Autodesk Inventor part; units mm, degrees
ref_plane "Work Plane1" through (0, -29.2355, 5.6836) normal (0, 0, 1) x (1, 0, 0)
ref_plane "Work Plane2" through (8.9574, 21.5645, 5.6836) normal (0.1736, 0.9848, 0) x (-0.9848, 0.1736, 0)
ref_plane "Work Plane3" through (-21.5633, 21.5645, 5.6836) normal (-0.3907, 0.9205, 0) x (-0.9205, -0.3907, 0)
sketch "Sketch1" plane through (0, 0, 0) normal (1, 0, 0) x (0, 1, 0)
  line L0 (9.6583, 12.5432) -> (9.6583, -1.1759)
  line L1 (9.6583, -1.1759) -> (4.0957, -1.1759)
  line L2 (4.0957, -1.1759) -> (4.0957, -6.5068)
  line L3 (4.0957, -6.5068) -> (-0.6541, -6.5068)
  line L4 (-0.6541, -6.5068) -> (-0.6541, 9.1142)
  line L5 (-0.6541, 9.1142) -> (-3.0417, 9.1142)
  line L6 (-3.0417, 9.1142) -> (-3.0417, 12.5432)
  line L7 (-3.0417, 12.5432) -> (9.6583, 12.5432)
  line L8 (9.6583, 12.5432) -> (-29.2355, 12.5432) construction
  line L9 (-29.2355, 12.5432) -> (-29.2355, -33.1187) construction
  point P0 (0, 0)
  dimension "d0" = 12.7
  dimension "d1" = 19.05
  dimension "d2" = 5.5626
  dimension "d3" = 10.3124
  dimension "d4" = 3.429
  dimension "d5" = 38.8937
revolve "Revolution1" add sketch "Sketch1" angle 360 about axis through (0, -29.2355, 12.5432) along (0, 0, -1)
chamfer "Chamfer1" distance 0.7874 angle 45 1 edges at (0, -62.5666, -6.5068)
sketch "Sketch2" plane through (0, -29.2355, 12.5432) normal (0, 0, 1) x (1, 0, 0)
  circle A0 centre (0, 0) radius 38.8938
  circle A1 centre (0, 0) radius 33.3312
  circle A2 centre (0, 33.3312) radius 3.175
  circle A3 centre (-28.8656, -16.6656) radius 3.175
  circle A4 centre (28.8656, -16.6656) radius 3.175
  point P0 (0, 29.2355)
  dimension "d10" = 6.35
  dimension "d13" = 360
extrude "Extrusion1" cut sketch "Sketch2" against normal blind 10.3124 contours A2 A1 | A1 A2 | A4 A1 | A1 A4 | A3 A1 | A1 A3
ref_plane "Work Plane1" through (0, -29.2355, 5.6836) normal (0, 0, 1) x (1, 0, 0)
sketch "Sketch4" plane through (0, -29.2355, 5.6836) normal (0, 0, 1) x (1, 0, 0)
  line L0 (0, 0) -> (0, 62.7832) construction
  circle A0 centre (0, 0) radius 28.5814
  line L1 (-11.1676, 26.3093) -> (-21.5633, 50.8)
  line L2 (4.9631, 28.1471) -> (8.9574, 50.8)
  point P0 (0, 29.2355)
  dimension "d21" = 23
  dimension "d22" = 10
  dimension "d23" = 50.8
  dimension "d24" = 50.8
ref_plane "Work Plane2" through (8.9574, 21.5645, 5.6836) normal (0.1736, 0.9848, 0) x (-0.9848, 0.1736, 0)
sketch "Sketch5" plane through (8.9574, 21.5645, 5.6836) normal (0.1736, 0.9848, 0) x (-0.9848, 0.1736, 0)
  circle A0 centre (0, 0) radius 2.54
  point P0 (5.0767, -5.6836)
  dimension "d25" = 5.08
extrude "Extrusion2" add sketch "Sketch5" against normal blind 20.6375
ref_plane "Work Plane3" through (-21.5633, 21.5645, 5.6836) normal (-0.3907, 0.9205, 0) x (-0.9205, -0.3907, 0)
sketch "Sketch7" plane through (-21.5633, 21.5645, 5.6836) normal (-0.3907, 0.9205, 0) x (-0.9205, -0.3907, 0)
  circle A0 centre (0, 0) radius 2.54
  point P0 (-11.4232, -5.6836)
  dimension "d28" = 5.08
extrude "Extrusion3" add sketch "Sketch7" against normal blind 20.6375
fillet "Fillet1" radius 1.5875 1 edges at (11.4588, 21.1235, 5.6836)
fillet "Fillet2" radius 1.5875 1 edges at (-19.2252, 22.557, 5.6836)
For this review, take the finished solid that the model builds, in its own axes (mm). A direction names the side the tool comes from. Round coordinates to 2 decimals unless told otherwise and drop trailing zeros. Loops run counter-clockwise (first coordinate to the right, second up) from the corner with the lowest first, then second, coordinate; pieces in that order, holes last. Notation, with made-up numbers: (16.25, 81.25) - (75.25, 81.25) arc R27 ccw to (75.25, 115.25) - close; hole circle Ø1 at (57, 72). An arc over 180 degrees is marked (long way). Use one line per item in the form item = value.
Item 1: For line 1 (Y direction, x = 13, z = -0.25); line 2 (X direction, y = -45, z = 0.75); line 3 (X direction, y = -53.5, z = 6.75), list the stretches that pass through material, from the lowest coordinate up.
Answers:
line_1 = -65.89 to -54.69, -3.78 to 7.42
line_2 = -35.56 to -23.84, 23.84 to 35.56
line_3 = -30.4 to -15.1, 15.1 to 30.4
Item 2: Consider section B-B on z = 0.25. Write out the cut boundary in (x, y).
Answers:
outline = circle Ø77.79 at (0, -29.24); hole circle Ø57.16 at (0, -29.24)
Item 3: Mouldability with a two-part tool opening along Y and no side actions: class faces 1 (the cylindrical face through (-0.413, 7.244, 7.459)), 2 (the cylindrical face through (10.012, 2.557, -3.479)), 3 (the flat face through (-25.4, -21.1, 12.543)) as +Y half, -Y half, draft (parallel to the pull), parting line (faces both ways), or undercut.
Answers:
face_1 = undercut
face_2 = parting line
face_3 = draft
Item 4: Consider section A-A on x = 0. Write out the cut boundary in (y, z).
Answers:
outline = (-68.13, -1.18) - (-62.57, -1.18) - (-62.57, -5.72) - (-61.78, -6.51) - (-57.82, -6.51) - (-57.82, 9.11) - (-55.43, 9.11) - (-55.43, 12.54) - (-68.13, 12.54) - close; (-3.04, 9.11) - (-0.65, 9.11) - (-0.65, -6.51) - (3.31, -6.51) - (4.1, -5.72) - (4.1, -1.18) - (9.66, -1.18) - (9.66, 12.54) - (7.27, 12.54) - (7.27, 2.23) - (0.92, 2.23) - (0.92, 12.54) - (-3.04, 12.54) - close
Item 5: Tool access review of faces 4 (the flat face through (0, 4, 2.231)), 5 (the cylindrical face through (-1.26, -57.79, 1.41)), 6 (the cylindrical face through (8.05, 14.51, 8.2)): name each direction out of +Z, -Z, +X, -X, +Y, -Y from which nothing blocks a thin tool from reaching the whole face with its end or side.
Answers:
face_4 = +Z
face_5 = -Z
face_6 = none
Item 6: Clearance check with flat-ended pins moving along their axes: P1, Ø4, axis at x = -29.5, z = -0.5, coming from the -Y side; P2, Ø2, axis at x = 5, y = 6, coming from the -Z side; P3, Ø6, axis at x = 11.5, z = 10.5, coming from the -Y side. State where each tip first meets the part, or that it passes through.
Answers:
P1 = -56.74
P2 = -1.18
P3 = -67.19
